Part model, mm, in its own coordinate system. A direction names the side the tool comes from. Round coordinates to 2 decimals unless told otherwise and drop trailing zeros. Write each loop counter-clockwise with the first axis right and the second up, starting at its lowest first coordinate (ties: lowest second). Pieces come first, ordered by that corner, then holes.
1) Drill centre lines: L1, parallel to Z at x = 190.5, y = 4.75; L2, parallel to X at y = 4, z = -132.5. Where is each one in solid material? Low to high.
2) Pull direction X, two halves, no side cores. Call faces 4 (the flat face through (177, 3, -218.65)), 5 (the flat face through (19, 3, -225)), 6 (the flat face through (218.65, 3, -80)), 7 (the flat face through (32.143, 3, -222)): +X half, -X half, draft (parallel to the pull), parting line (faces both ways), or undercut.
3) Saw through at A-A on z = -15.5. Write the cut outline in (x, y), and give its area (3 significant figures).
4) Flat gauge pins, fed straight in: pin 1 (1.9 mm diameter, centred on x = 221.5, y = 4.5, fed in from +Z); pin 2 (3 mm diameter, centred on y = 2, z = -85.5, fed in from +X); pin 3 (3 mm diameter, centred on y = 3.5, z = -201.5, fed in from +X). Where does each tip first touch, or does it go through?
5) Which spindle directions (+Z, -Z, +X, -X, +Y, -Y) get a long thin tool onto all of the face, cutting with end or side? Do faces 1 (the flat face through (3, 3, -160.714)), 2 (the flat face through (32.143, 3, -3)), 3 (the flat face through (218.65, 3, -16)). Say none if no direction does.
6) Saw through at B-B on x = 104. Write the cut outline in (y, z), and give its area (3 significant figures).
```python
from build123d import *

# Parameters (mm, degrees)
SKETCH1_W           = 6.35
SKETCH1_H           = 32.142857142
SKETCH1_H_2         = 32.142857143
SKETCH1_W_2         = 25.792857143
SKETCH1_H_3         = 6.35
SKETCH1_W_3         = 32.142857143
BOSS_EXTRUDE1_DEPTH = 6.35


with BuildPart() as part:
    # Sketch1 → Boss-Extrude1 (new body)
    with BuildSketch(Plane(origin=(0, 0, 0), x_dir=(1, 0, 0), z_dir=(0, 1, 0))):
        Polygon((6.35, 6.35), (32.142857143, 6.35), (64.285714286, 6.35), (96.428571429, 6.35), (128.571428571, 6.35), (160.714285714, 6.35), (192.857142857, 6.35), (218.65, 6.35), (218.65, 32.142857143), (218.65, 64.285714286), (218.65, 96.428571429), (218.65, 128.571428571), (218.65, 160.714285714), (218.65, 192.857142857), (218.65, 218.65), (192.857142857, 218.65), (160.714285714, 218.65), (128.571428571, 218.65), (96.428571429, 218.65), (64.285714286, 218.65), (32.142857143, 218.65), (6.35, 218.65), (6.35, 192.857142857), (6.35, 160.714285714), (6.35, 128.571428571), (6.35, 96.428571429), (6.35, 64.285714286), (6.35, 32.142857143), align=None)
        with Locations((3.175, 112.5)):
            Rectangle(SKETCH1_W, SKETCH1_H)
        with Locations((3.175, 48.214285715)):
            Rectangle(SKETCH1_W, SKETCH1_H_2)
        with Locations((3.175, 176.785714286)):
            Rectangle(SKETCH1_W, SKETCH1_H_2)
        with Locations((19.246428572, 3.175)):
            Rectangle(SKETCH1_W_2, SKETCH1_H_3)
        with Locations((80.357142858, 3.175)):
            Rectangle(SKETCH1_W_3, SKETCH1_H_3)
        with Locations((144.642857143, 3.175)):
            Rectangle(SKETCH1_W_3, SKETCH1_H_3)
        with Locations((205.753571429, 3.175)):
            Rectangle(SKETCH1_W_2, SKETCH1_H_3)
        with Locations((221.825, 48.214285715)):
            Rectangle(SKETCH1_W, SKETCH1_H_2)
        with Locations((221.825, 112.5)):
            Rectangle(SKETCH1_W, SKETCH1_H)
        with Locations((221.825, 176.785714286)):
            Rectangle(SKETCH1_W, SKETCH1_H_2)
        with Locations((205.753571429, 221.825)):
            Rectangle(SKETCH1_W_2, SKETCH1_H_3)
        with Locations((144.642857143, 221.825)):
            Rectangle(SKETCH1_W_3, SKETCH1_H_3)
        with Locations((80.357142858, 221.825)):
            Rectangle(SKETCH1_W_3, SKETCH1_H_3)
        with Locations((19.246428572, 221.825)):
            Rectangle(SKETCH1_W_2, SKETCH1_H_3)
    extrude(amount=BOSS_EXTRUDE1_DEPTH)


solid = part.part
```
Completed:
1. L1: z = -218.65 to -6.35
1. L2: x = 6.35 to 218.65
2. face 4: undercut
2. face 5: draft
2. face 6: +X half
2. face 7: undercut
3. outline: (6.35, 0) - (218.65, 0) - (218.65, 6.35) - (6.35, 6.35) - close
3. area: 1,350 mm2
4. pin 1: stops at z = -32.14
4. pin 2: stops at x = 218.65
4. pin 3: stops at x = 218.65
5. face 1: -X, +Y, -Y
5. face 2: +Z, +Y, -Y
5. face 3: +Z, +X, +Y, -Y
6. outline: (0, -218.65) - (6.35, -218.65) - (6.35, -6.35) - (0, -6.35) - close
6. area: 1,350 mm2
